from build123d import *

# Parameters (mm, degrees)
F0_R     = 2
F1_DEPTH = 9


with BuildPart() as f1:
    # F0 (on Front) → F1 (new body)
    with BuildSketch(Plane.XZ):
        Polygon((265.897079, -111.097285), (265.897079, 120.763555), (212.761675, 120.763555), (212.761675, 198.045397), (174.114259, 198.045397), (174.114259, 246.352586), (82.3411, 246.352586), (82.3411, 285.000002), (-130.196029, 285.000002), (-130.196029, 246.352586), (-217.152296, 246.352586), (-217.152296, 198.045397), (-265.461152, 198.045397), (-265.461152, 120.763555), (-182.215667, 120.657777), (-182.292131, 78.99439), (-40.622253, 80.756165), (-39.717878, 37.151925), (50.208882, 36.247385), (51.121586, -25.518982), (-39.717878, -26.429854), (-39.717878, -70.935305), (-180.510698, -71.846343), (-180.510698, -115.447249), (-265.897079, -116.364784), (-265.461152, -183.560564), (-217.152296, -183.560564), (-217.152296, -246.360741), (-130.196029, -246.360741), (-130.196029, -284.999998), (82.3411, -284.999998), (82.3411, -246.360741), (174.114259, -246.360741), (174.114259, -183.560564), (212.761675, -183.560564), (212.761675, -111.097285), align=None)
        with Locations((-169.174156, -241.860734)):
            Circle(F0_R, mode=Mode.SUBTRACT)
        with Locations((-236.821267, -179.060557)):
            Circle(F0_R, mode=Mode.SUBTRACT)
        with Locations((-212.652289, -210.460646)):
            Circle(F0_R, mode=Mode.SUBTRACT)
        with Locations((-261.179171, -149.93847)):
            Circle(F0_R, mode=Mode.SUBTRACT)
        with Locations((-125.696022, -261.180363)):
            Circle(F0_R, mode=Mode.SUBTRACT)
        with Locations((-23.927464, -280.499991)):
            Circle(F0_R, mode=Mode.SUBTRACT)
        with Locations((-218.689395, -120.357772)):
            Circle(F0_R, mode=Mode.SUBTRACT)
        with Locations((-176.010692, -98.108243)):
            Circle(F0_R, mode=Mode.SUBTRACT)
        with Locations((-105.614282, -75.861807)):
            Circle(F0_R, mode=Mode.SUBTRACT)
        with Locations((-35.217872, -53.145626)):
            Circle(F0_R, mode=Mode.SUBTRACT)
        with Locations((77.841094, -261.180363)):
            Circle(F0_R, mode=Mode.SUBTRACT)
        with Locations((123.727673, -241.860734)):
            Circle(F0_R, mode=Mode.SUBTRACT)
        with Locations((169.614252, -210.460646)):
            Circle(F0_R, mode=Mode.SUBTRACT)
        with Locations((188.937961, -179.060557)):
            Circle(F0_R, mode=Mode.SUBTRACT)
        with Locations((208.261669, -142.828918)):
            Circle(F0_R, mode=Mode.SUBTRACT)
        with Locations((10.235017, -30.429196)):
            Circle(F0_R, mode=Mode.SUBTRACT)
        with Locations((234.829371, -106.597278)):
            Circle(F0_R, mode=Mode.SUBTRACT)
        with Locations((-219.334275, 125.204953)):
            Circle(F0_R, mode=Mode.SUBTRACT)
        with Locations((-177.74558, 104.351434)):
            Circle(F0_R, mode=Mode.SUBTRACT)
        with Locations((-35.762538, 63.459567)):
            Circle(F0_R, mode=Mode.SUBTRACT)
        with Locations((-106.999755, 84.431064)):
            Circle(F0_R, mode=Mode.SUBTRACT)
        with Locations((-260.961145, 159.401619)):
            Circle(F0_R, mode=Mode.SUBTRACT)
        with Locations((-236.806717, 193.54539)):
            Circle(F0_R, mode=Mode.SUBTRACT)
        with Locations((-212.652289, 217.698985)):
            Circle(F0_R, mode=Mode.SUBTRACT)
        with Locations((-169.174156, 241.852579)):
            Circle(F0_R, mode=Mode.SUBTRACT)
        with Locations((-125.696022, 261.176288)):
            Circle(F0_R, mode=Mode.SUBTRACT)
        with Locations((-23.927464, 280.499996)):
            Circle(F0_R, mode=Mode.SUBTRACT)
        with Locations((55.165724, 5.364793)):
            Circle(F0_R, mode=Mode.SUBTRACT)
        with Locations((9.66711, 41.155414)):
            Circle(F0_R, mode=Mode.SUBTRACT)
        with Locations((261.397073, 4.833135)):
            Circle(F0_R, mode=Mode.SUBTRACT)
        with Locations((234.829371, 116.263548)):
            Circle(F0_R, mode=Mode.SUBTRACT)
        with Locations((123.727673, 241.852579)):
            Circle(F0_R, mode=Mode.SUBTRACT)
        with Locations((77.841094, 261.176288)):
            Circle(F0_R, mode=Mode.SUBTRACT)
        with Locations((188.937961, 193.54539)):
            Circle(F0_R, mode=Mode.SUBTRACT)
        with Locations((208.261669, 154.904469)):
            Circle(F0_R, mode=Mode.SUBTRACT)
        with Locations((169.614252, 217.698985)):
            Circle(F0_R, mode=Mode.SUBTRACT)
    extrude(amount=F1_DEPTH)


solid = f1.part
Could you check a few things on this model? Use its own coordinates, in mm. Give positions to 0.01 mm unless a question says otherwise; leave off trailing zeros. Order: outer loops, then holes, each group sorted by start corner. A loop starts at its lowest first (then second) coordinate and runs counter-clockwise, first axis right, second up. Notation, with made-up numbers: (88.5, 63) - (127.5, 63) arc R21 cw to (127.5, 74) - close; hole circle Ø3 at (73, -34). An arc over 180 degrees is marked (long way). Return JSON: item names as keys, results as strings. Group by question number.
Q1. Suppose I cut it at C-C, the plane z = -166.5. Please give me the cut outline in (x, y).
Q2. Suppose I cut it at B-B, the plane x = -76. Please give me the cut outline in (y, z).
Q3. Suppose I cut it at A-A, the plane x = -2.5. Please give me the cut outline in (y, z), and give its area (3 significant figures).
Q4. Please list where these lines run through material, in increasing order: line 1 along Z through (x, y) = (-47, -3.25); line 2 along X through (y, z) = (-1.5, -241.5); line 3 along X through (y, z) = (-7.25, 84.5). Write a range as [from, to].
Q5. Suppose I cut it at D-D, the plane y = -7.25. State how many separate pieces and enclosed holes the cut face has, and give its area (3 significant figures).
Q6. Will these pins go through, and if not, where does the flat tip stop? pin 1 Ø5 at (y, z) = (-4.5, 217.5) entering from +X; pin 2 Ø3 at (x, y) = (-198, -5) entering from -Z; pin 3 Ø3 at (y, z) = (-5.5, 7) entering from -X.
Resolved:
{
 "1": {"outline": "(-265.57, -9) - (212.76, -9) - (212.76, 0) - (-265.57, 0) - close"},
 "2": {"outline": "(-9, -285) - (0, -285) - (0, -71.17) - (-9, -71.17) - close; (-9, 80.32) - (0, 80.32) - (0, 285) - (-9, 285) - close"},
 "3": {"outline": "(-9, -285) - (0, -285) - (0, -26.06) - (-9, -26.06) - close; (-9, 36.78) - (0, 36.78) - (0, 285) - (-9, 285) - close", "area": "4,560 mm2"},
 "4": {"line 1": "z = [-285, -70.98], [80.68, 285]", "line 2": "x = [-217.15, -171.14], [-167.21, 121.76], [125.69, 174.11]", "line 3": "x = [-182.28, -109], [-105, 265.9]"},
 "5": {"separate pieces": "1", "enclosed holes": "36", "area": "207,000 mm2"},
 "6": {"pin 1": "stops at x = 174.11", "pin 2": "stops at z = -246.36", "pin 3": "stops at x = 50.62"}
}
